Job drawing, mm, ordinate dimensions from the low corner. One solid piece. A direction names the side the tool comes from. Round coordinates to 2 decimals unless told otherwise and drop trailing zeros. Loops run counter-clockwise (first coordinate to the right, second up) from the corner with the lowest first, then second, coordinate; pieces in that order, holes last.
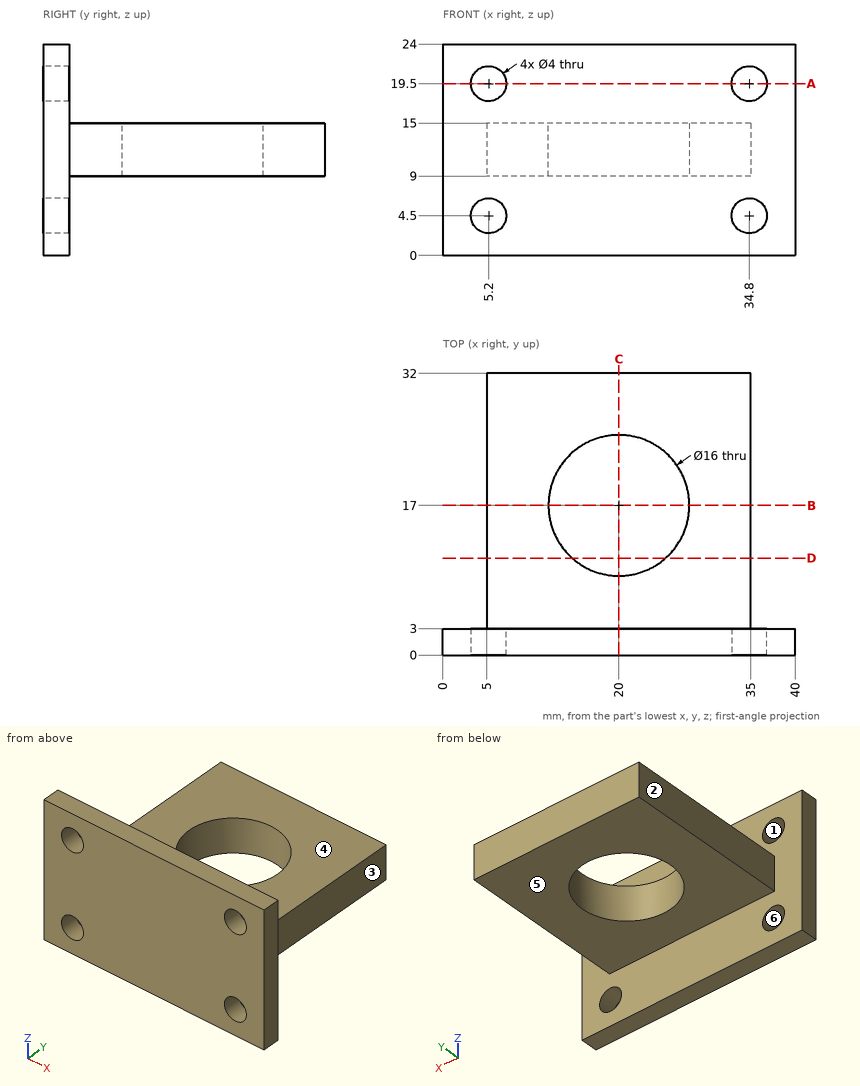
Item 1: Cut at D-D, the plane y = 11. Give the cut face in (x, z).
Answers follow:
outline: (5, 9) - (14.71, 9) - (14.71, 15) - (5, 15) - close; (25.29, 9) - (35, 9) - (35, 15) - (25.29, 15) - close
Item 2: Cut at B-B, the plane y = 17. Give the cut face in (x, z).
Answers follow:
outline: (5, 9) - (12, 9) - (12, 15) - (5, 15) - close; (28, 9) - (35, 9) - (35, 15) - (28, 15) - close
Item 3: Probe line 1 (Z direction, x = 5.2, y = 0.6); line 2 (X direction, y = 0.7, z = 19.5); line 3 (Z direction, x = 15, y = 5). List the from-to ranges inside material, lowest first.
Answers follow:
line 1: z = 0 to 2.5, 6.5 to 17.5, 21.5 to 24
line 2: x = 0 to 3.2, 7.2 to 32.8, 36.8 to 40
line 3: z = 9 to 15
Item 4: Two-plate mould, pull along Z, no slides. Class the marked faces 3, 4, 5 and 6: released by +Z, released by -Z, zero draft, split by the parting line, or undercut.
Answers follow:
face 3: zero draft
face 4: released by +Z
face 5: released by -Z
face 6: undercut
Item 5: Cut at C-C, the plane x = 20. Give the cut face in (y, z), plus the area to 3 significant figures.
Answers follow:
outline: (0, 0) - (3, 0) - (3, 9) - (9, 9) - (9, 15) - (3, 15) - (3, 24) - (0, 24) - close; (25, 9) - (32, 9) - (32, 15) - (25, 15) - close
area: 150 mm2
Item 6: 3-axis set-ups, long thin cutter, end or side, ignore diameter. For the marked faces 1 and 2: which of +Z, -Z, +X, -X, +Y, -Y reach the whole face in a straight line?
Answers follow:
face 1: +Y, -Y
face 2: +Z, -Z, -X, +Y
Item 7: Flat gauge pins, fed straight in: P1, Ø6, axis at x = 26, y = 26.5, coming from the +Z side; P2, Ø6.5, axis at y = 23, z = 11, coming from the -X side; P3, Ø4, axis at x = 18.5, z = 6, coming from the +Y side. Where does each tip first touch, or does it go through?
Answers follow:
P1: stops at z = 15
P2: stops at x = 5
P3: stops at y = 3
Item 8: Cut at A-A, the plane z = 19.5. Give the cut face in (x, y), plus the area to 3 significant figures.
Answers follow:
outline: (0, 0) - (3.2, 0) - (3.2, 3) - (0, 3) - close; (7.2, 0) - (32.8, 0) - (32.8, 3) - (7.2, 3) - close; (36.8, 0) - (40, 0) - (40, 3) - (36.8, 3) - close
area: 96.0 mm2
